The model under review builds one solid part; all positions refer to its coordinate system, in mm. Give positions to 0.01 mm unless a question says otherwise; leave off trailing zeros. Order: outer loops, then holes, each group sorted by start corner. A loop starts at its lowest first (then second) coordinate and runs counter-clockwise, first axis right, second up. Notation, with made-up numbers: (1.5, 85.5) - (45.5, 85.5) arc R17 cw to (45.5, 118.5) - close; hole circle Ø9 at (-29, 2). An arc over 180 degrees is marked (long way). Answer as CSV lines item,"result". Start each with the question number.
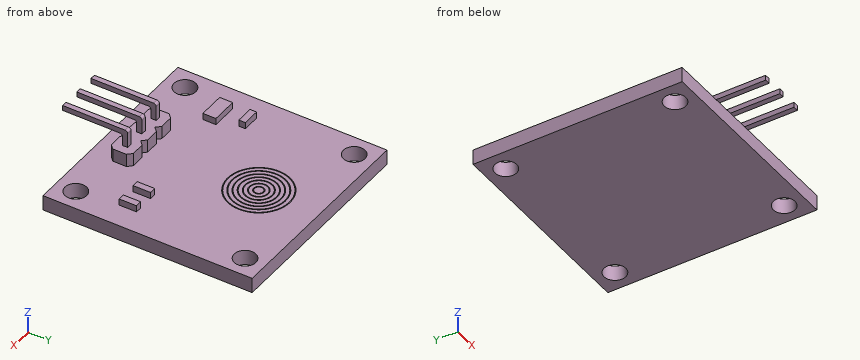
from build123d import *

# Parameters (mm, degrees)
SKETCH_W            = 24.1
SKETCH_H            = 24.1
PAD_DEPTH           = 1.75
SKETCH001_R         = 1.25
POCKET_DEPTH        = 1.751
PAD001_DEPTH        = 1.5
PAD002_DEPTH        = 0.3
PAD002_DEPTH_BACK   = 0.3
LINEARPATTERN_COUNT = 3
LINEARPATTERN_PITCH = 2.54
SKETCH005_W         = 0.75
SKETCH005_H         = 2
SKETCH005_W_2       = 3
SKETCH005_H_2       = 1.5
SKETCH005_W_3       = 2
SKETCH005_H_3       = 0.75
PAD003_DEPTH        = 0.75
SKETCH006_R         = 0.6
SKETCH006_R_2       = 0.5
POCKET001_DEPTH     = 0.25
SKETCH007_R         = 1.1
SKETCH007_R_2       = 1
POCKET002_DEPTH     = 0.25
SKETCH008_R         = 1.6
SKETCH008_R_2       = 1.5
POCKET003_DEPTH     = 0.25
SKETCH009_R         = 2.1
SKETCH009_R_2       = 2
POCKET004_DEPTH     = 0.25
SKETCH010_R         = 2.6
SKETCH010_R_2       = 2.5
POCKET005_DEPTH     = 0.25
SKETCH011_R         = 3.1
SKETCH011_R_2       = 3
POCKET006_DEPTH     = 0.25
SKETCH012_R         = 3.6
SKETCH012_R_2       = 3.5
POCKET007_DEPTH     = 0.25


with BuildPart() as part:
    # Sketch → Pad (new body)
    with BuildSketch(Plane.XY):
        Rectangle(SKETCH_W, SKETCH_H)
    extrude(amount=PAD_DEPTH)

    # Sketch001 (on Face6 of Pad) → Pocket (cut, through all)
    with BuildSketch(Plane.XY.offset(1.75)):
        with Locations((-9.75, 9.75)):
            Circle(SKETCH001_R)
        with Locations((9.75, 9.75)):
            Circle(SKETCH001_R)
        with Locations((-9.75, -9.75)):
            Circle(SKETCH001_R)
        with Locations((9.75, -9.75)):
            Circle(SKETCH001_R)
    extrude(amount=-POCKET_DEPTH, mode=Mode.SUBTRACT)

    # Sketch002 (on Face5 of Pocket) → Pad001 (join)
    with BuildSketch(Plane.XY.offset(1.75)):
        Polygon((-3.81, -7.744125), (-3.81, -9.315875), (-3.325875, -9.8), (-1.754125, -9.8), (-1.27, -9.315875), (-1.27, -7.744125), (-1.754125, -7.26), (-3.325875, -7.26), align=None)
    pad001 = extrude(amount=PAD001_DEPTH)

    # Sketch004 (on DatumPlane) → Pad002 (join, two sides)
    with BuildSketch(Plane.YZ.offset(-2.54)) as pad002_sk:
        with BuildLine():
            Line((-8.83, 3.25), (-8.23, 3.25))
            Line((-8.23, 3.25), (-8.23, 4.95))
            ThreePointArc((-8.23, 4.95), (-8.317868, 5.162132), (-8.53, 5.25))
            Line((-8.53, 5.25), (-15.73, 5.25))
            Line((-15.73, 5.25), (-15.73, 4.65))
            Line((-15.73, 4.65), (-9.13, 4.65))
            ThreePointArc((-8.83, 4.35), (-8.917868, 4.562132), (-9.13, 4.65))
            Line((-8.83, 4.35), (-8.83, 3.25))
        make_face()
    pad002 = extrude(amount=PAD002_DEPTH) + extrude(pad002_sk.sketch, amount=-PAD002_DEPTH_BACK)

    # LinearPattern: Pad002, Pad001 ×3
    with Locations(*[(i * LINEARPATTERN_PITCH, 0, 0) for i in range(1, LINEARPATTERN_COUNT)]):
        add(pad002)
        add(pad001)

    # Sketch005 (on Face5 of LinearPattern) → Pad003 (join)
    with BuildSketch(Plane.XY.offset(1.75)):
        with Locations((8.925, -4.05)):
            Rectangle(SKETCH005_W, SKETCH005_H)
        with Locations((6.425, -4.05)):
            Rectangle(SKETCH005_W, SKETCH005_H)
        with Locations((-7.95, -4.8)):
            Rectangle(SKETCH005_W_2, SKETCH005_H_2)
        with Locations((-8.45, -1.675)):
            Rectangle(SKETCH005_W_3, SKETCH005_H_3)
    extrude(amount=PAD003_DEPTH)

    # Sketch006 (on Face5 of Pad003) → Pocket001 (cut)
    with BuildSketch(Plane.XY.offset(1.75)):
        with Locations((0, 5.05)):
            Circle(SKETCH006_R)
        with Locations((0, 5.05)):
            Circle(SKETCH006_R_2, mode=Mode.SUBTRACT)
    extrude(amount=-POCKET001_DEPTH, mode=Mode.SUBTRACT)

    # Sketch007 (on Face5 of Pocket001) → Pocket002 (cut)
    with BuildSketch(Plane.XY.offset(1.75)):
        with Locations((0, 5.05)):
            Circle(SKETCH007_R)
        with Locations((0, 5.05)):
            Circle(SKETCH007_R_2, mode=Mode.SUBTRACT)
    extrude(amount=-POCKET002_DEPTH, mode=Mode.SUBTRACT)

    # Sketch008 (on Face5 of Pocket002) → Pocket003 (cut)
    with BuildSketch(Plane.XY.offset(1.75)):
        with Locations((0, 5.05)):
            Circle(SKETCH008_R)
        with Locations((0, 5.05)):
            Circle(SKETCH008_R_2, mode=Mode.SUBTRACT)
    extrude(amount=-POCKET003_DEPTH, mode=Mode.SUBTRACT)

    # Sketch009 (on Face5 of Pocket003) → Pocket004 (cut)
    with BuildSketch(Plane.XY.offset(1.75)):
        with Locations((0, 5.05)):
            Circle(SKETCH009_R)
        with Locations((0, 5.05)):
            Circle(SKETCH009_R_2, mode=Mode.SUBTRACT)
    extrude(amount=-POCKET004_DEPTH, mode=Mode.SUBTRACT)

    # Sketch010 (on Face5 of Pocket004) → Pocket005 (cut)
    with BuildSketch(Plane.XY.offset(1.75)):
        with Locations((0, 5.05)):
            Circle(SKETCH010_R)
        with Locations((0, 5.05)):
            Circle(SKETCH010_R_2, mode=Mode.SUBTRACT)
    extrude(amount=-POCKET005_DEPTH, mode=Mode.SUBTRACT)

    # Sketch011 (on Face5 of Pocket005) → Pocket006 (cut)
    with BuildSketch(Plane.XY.offset(1.75)):
        with Locations((0, 5.05)):
            Circle(SKETCH011_R)
        with Locations((0, 5.05)):
            Circle(SKETCH011_R_2, mode=Mode.SUBTRACT)
    extrude(amount=-POCKET006_DEPTH, mode=Mode.SUBTRACT)

    # Sketch012 (on Face5 of Pocket006) → Pocket007 (cut)
    with BuildSketch(Plane.XY.offset(1.75)):
        with Locations((0, 5.05)):
            Circle(SKETCH012_R)
        with Locations((0, 5.05)):
            Circle(SKETCH012_R_2, mode=Mode.SUBTRACT)
    extrude(amount=-POCKET007_DEPTH, mode=Mode.SUBTRACT)


solid = part.part
Item 1: Take a section at D-D on y = -3.5. Write out the cut boundary in (x, z), and give its area (3 significant figures).
Item 2: For line 1 along Z through (x, y) = (-1.75, -9.5); line 2 along Y through (x, z) = (6.75, 0.65); line 3 along Z through (x, y) = (2.5, 3), list the stretches that pass through material, from the lowest coordinate up.
Item 3: Take a section at A-A on x = 9.75. Write out the cut boundary in (y, z).
Item 4: Clearance check with flat-ended pins moving along their axes: pin 1 (5 mm diameter, centred on x = -3, y = -5, fed in from +Z); pin 2 (0.8 mm diameter, centred on x = -8.5, y = -5, fed in from +Z); pin 3 (1 mm diameter, centred on y = -12, z = 3, fed in from +X); pin 4 (2.5 mm diameter, centred on x = 1, y = 6.5, fed in from +Z). State where each tip first meets the part, or that it passes through.
Item 5: Take a section at B-B on y = -13.5. Write out the cut boundary in (x, z), and give its area (3 significant figures).
Item 6: Take a section at C-C on x = -8. Write out the cut boundary in (y, z).
Data:
1,outline,"(-12.05, 0) - (12.05, 0) - (12.05, 1.75) - (9.3, 1.75) - (9.3, 2.5) - (8.55, 2.5) - (8.55, 1.75) - (6.8, 1.75) - (6.8, 2.5) - (6.05, 2.5) - (6.05, 1.75) - (-12.05, 1.75) - close"
1,area,"43.3 mm^2"
2,line 1,"z = 0 to 3.25"
2,line 2,"y = -12.05 to 12.05"
2,line 3,"z = 0 to 1.75"
3,outline,"(-12.05, 0) - (-11, 0) - (-11, 1.75) - (-12.05, 1.75) - close; (-8.5, 0) - (8.5, 0) - (8.5, 1.75) - (-8.5, 1.75) - close; (11, 0) - (12.05, 0) - (12.05, 1.75) - (11, 1.75) - close"
4,pin 1,"stops at z = 3.25"
4,pin 2,"stops at z = 2.5"
4,pin 3,"passes through"
4,pin 4,"stops at z = 1.75"
5,outline,"(-2.84, 4.65) - (-2.24, 4.65) - (-2.24, 5.25) - (-2.84, 5.25) - close; (-0.3, 4.65) - (0.3, 4.65) - (0.3, 5.25) - (-0.3, 5.25) - close; (2.24, 4.65) - (2.84, 4.65) - (2.84, 5.25) - (2.24, 5.25) - close"
5,area,"1.08 mm^2"
6,outline,"(-12.05, 0) - (12.05, 0) - (12.05, 1.75) - (-1.3, 1.75) - (-1.3, 2.5) - (-2.05, 2.5) - (-2.05, 1.75) - (-4.05, 1.75) - (-4.05, 2.5) - (-5.55, 2.5) - (-5.55, 1.75) - (-12.05, 1.75) - close"
